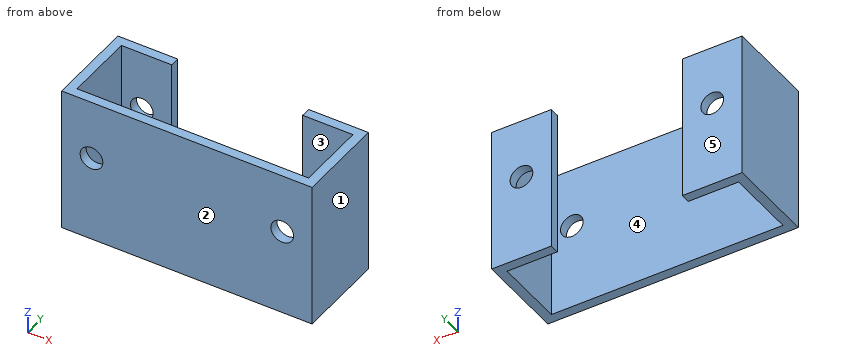
```python
from build123d import *

# Parameters (mm, degrees)
BOSS_EXTRUDE1_START   = -14.5
BOSS_EXTRUDE1_DEPTH   = 24.5
F_6_CLEARANCE_HOLE1_D = 3.7973


with BuildPart() as part:
    # Sketch1 → Boss-Extrude1 (new body)
    with BuildSketch(Plane.XY.offset(BOSS_EXTRUDE1_START)):
        Polygon((20.965, 0), (0, 0), (0, 15), (10, 15), (10, 13.4125), (1.5875, 13.4125), (1.5875, 1.5875), (20.965, 1.5875), align=None)
    boss_extrude1 = extrude(amount=BOSS_EXTRUDE1_DEPTH)

    # #6 Clearance Hole1 (through all)
    with Locations(Plane(origin=(0, 0, 0), x_dir=(-1, 0, 0), z_dir=(0, -1, 0))):
        with Locations((-5, 0)):
            f_6_clearance_hole1 = Hole(F_6_CLEARANCE_HOLE1_D / 2)

    # Mirror1: Boss-Extrude1, #6 Clearance Hole1 across plane
    add(boss_extrude1.mirror(Plane(origin=(20.965, 1.5875, -14.5), x_dir=(0, 0, 1), z_dir=(1, 0, 0))))
    add(f_6_clearance_hole1.mirror(Plane(origin=(20.965, 1.5875, -14.5), x_dir=(0, 0, 1), z_dir=(1, 0, 0))), mode=Mode.SUBTRACT)


solid = part.part
```
Geometry check sheet. Reference: the model listing, model coordinates, mm. Face numbers are marked on the shaded views. A direction names the side the tool comes from. Coordinates: 2 decimals unless noted, no trailing zeros. Order: outer loops, then holes, each group sorted by start corner. A loop starts at its lowest first (then second) coordinate and runs counter-clockwise, first axis right, second up. Notation, with made-up numbers: M 21.5,-26.5 L 30.5,-26.5 A18 ccw 30.5,-18.5 Z; hole C 33,47.25 d8. An arc over 180 degrees is marked long. One line per question, with ' | ' between items. Start each with the question number.
Item 1: Draft check along X on the marked faces 1, 2 and 3. Enter one of: pulls with the +X half, pulls with the -X half, needs draft (parallel to the pull), parting line crosses it, or undercut.
Item 2: Cross-section at C-C on z = 0. Enter the section's corners in (x, y), then the cut area to 3 significant figures.
Item 3: Cross-section at D-D on x = 21.5. Enter the section's corners in (y, z).
Item 4: Cross-section at A-A on x = 36.93. Enter the section's corners in (y, z), then the cut area to 3 significant figures.
Item 5: Gauge pin test, flat ends, axial feed: pin 1 (0.8 mm diameter, centred on y = 14, z = -5, fed in from -X); pin 2 (3.5 mm diameter, centred on x = 5, z = 0, fed in from -Y). Record the tip position at first contact, or that the pin passes through.
Item 6: Set-up check for the marked faces 4 and 5: record each of +Z, -Z, +X, -X, +Y, -Y from which the full face is reachable in a straight line by a thin tool's end or side.
Item 7: Cross-section at B-B on y = 4.5. Enter the section's corners in (x, z), then the cut area to 3 significant figures.
Item 8: Material ranges on L1, parallel to X at y = 12, z = 4.5; L2, parallel to Z at x = 36.93, y = 0.7; L3, parallel to Y at x = 39.5, z = -9.5, recorded low to high. Write a range as [from, to].
Findings:
1) face 1: pulls with the +X half | face 2: needs draft | face 3: undercut
2) outline: M 0,0 L 3.1,0 L 3.1,1.59 L 1.59,1.59 L 1.59,13.41 L 3.1,13.41 L 3.1,15 L 0,15 Z; M 6.9,0 L 35.03,0 L 35.03,1.59 L 6.9,1.59 Z; M 6.9,13.41 L 10,13.41 L 10,15 L 6.9,15 Z; M 31.93,13.41 L 35.03,13.41 L 35.03,15 L 31.93,15 Z; M 38.83,0 L 41.93,0 L 41.93,15 L 38.83,15 L 38.83,13.41 L 40.34,13.41 L 40.34,1.59 L 38.83,1.59 Z | area: 112 mm²
3) outline: M 0,-14.5 L 1.59,-14.5 L 1.59,10 L 0,10 Z
4) outline: M 0,-14.5 L 1.59,-14.5 L 1.59,-1.9 L 0,-1.9 Z; M 0,1.9 L 1.59,1.9 L 1.59,10 L 0,10 Z; M 13.41,-14.5 L 15,-14.5 L 15,-1.9 L 13.41,-1.9 Z; M 13.41,1.9 L 15,1.9 L 15,10 L 13.41,10 Z | area: 65.7 mm²
5) pin 1: stops at x = 0 | pin 2: passes through
6) face 4: +Z, -Z | face 5: +Z, -Z, +X, -X, +Y
7) outline: M 0,-14.5 L 1.59,-14.5 L 1.59,10 L 0,10 Z; M 40.34,-14.5 L 41.93,-14.5 L 41.93,10 L 40.34,10 Z | area: 77.8 mm²
8) L1: x = [0, 1.59], [40.34, 41.93] | L2: z = [-14.5, -1.9], [1.9, 10] | L3: y = [0, 1.59], [13.41, 15]
